Part print with two shaded views. Sizes in mm from the minimum x, y, z corner. A direction names the side the tool comes from. Round coordinates to 2 decimals unless told otherwise and drop trailing zeros. Loops run counter-clockwise (first coordinate to the right, second up) from the corner with the lowest first, then second, coordinate; pieces in that order, holes last. Notation, with made-up numbers: (-6.75, -35.75) -> (28.25, -35.75) arc R34 cw to (28.25, -0.75) -> close; hole circle Ø3 at (-10.5, -37). An arc over 180 degrees is marked (long way). Answer as a JSON object with one key per item and string values. Group by question number.
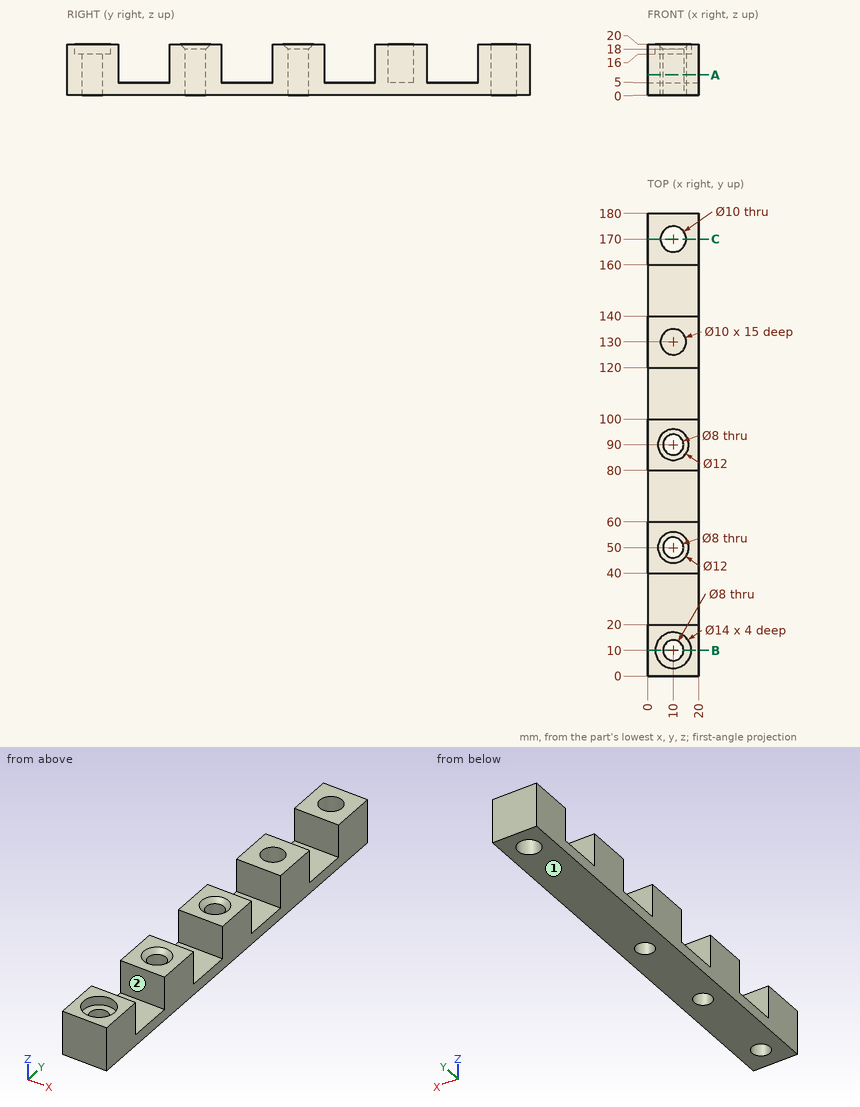
Item 1: Band-saw the part on A-A, the plane z = 8. Count the separate pieces of the cut face and the enclosed holes in it, plus the area to 3 significant figures.
Item 2: Which spindle directions (+Z, -Z, +X, -X, +Y, -Y) get a long thin tool onto all of the face, cutting with end or side? Do the marked faces 1 and 2. Say none if no direction does.
Item 3: Drill centre lines: line 1 (Y direction, x = 17.25, z = 12.25); line 2 (Y direction, x = 8, z = 4.25); line 3 (Z direction, x = 8.75, y = 78). Where is each one in solid material? Low to high.
Item 4: Band-saw the part on C-C, the plane y = 170. List the corners of the cut face in (x, z).
Item 5: Drop flat-ended pins along their axis: pin 1 Ø8 at (x, y) = (10, 130) entering from +Z; pin 2 Ø9 at (x, y) = (10, 10) entering from +Z. Give the stop position or say it passes through.
Item 6: Band-saw the part on B-B, the plane y = 10. List the corners of the cut face in (x, z), plus the area to 3 significant figures.
Entries:
{
 "1": {"separate pieces": "5", "enclosed holes": "5", "area": "1,690 mm²"},
 "2": {"face 1": "-Z, +X, -X, +Y, -Y", "face 2": "+Z, +X, -X"},
 "3": {"line 1": "0 to 20, 40 to 60, 80 to 100, 120 to 140, 160 to 180", "line 2": "0 to 6.54, 13.46 to 46.54, 53.46 to 86.54, 93.46 to 165.42, 174.58 to 180", "line 3": "0 to 5"},
 "4": {"outline": "(0, 0) -> (5, 0) -> (5, 20) -> (0, 20) -> close; (15, 0) -> (20, 0) -> (20, 20) -> (15, 20) -> close"},
 "5": {"pin 1": "z = 5", "pin 2": "z = 16"},
 "6": {"outline": "(0, 0) -> (6, 0) -> (6, 16) -> (3, 16) -> (3, 20) -> (0, 20) -> close; (14, 0) -> (20, 0) -> (20, 20) -> (17, 20) -> (17, 16) -> (14, 16) -> close", "area": "216 mm²"}
}
